Check sheet for the drawn part. Datum: minimum x, y, z corner. Units: mm. A direction names the side the tool comes from. Give positions to 0.01 mm unless a question says otherwise; leave off trailing zeros. Order: outer loops, then holes, each group sorted by start corner. A loop starts at its lowest first (then second) coordinate and runs counter-clockwise, first axis right, second up.
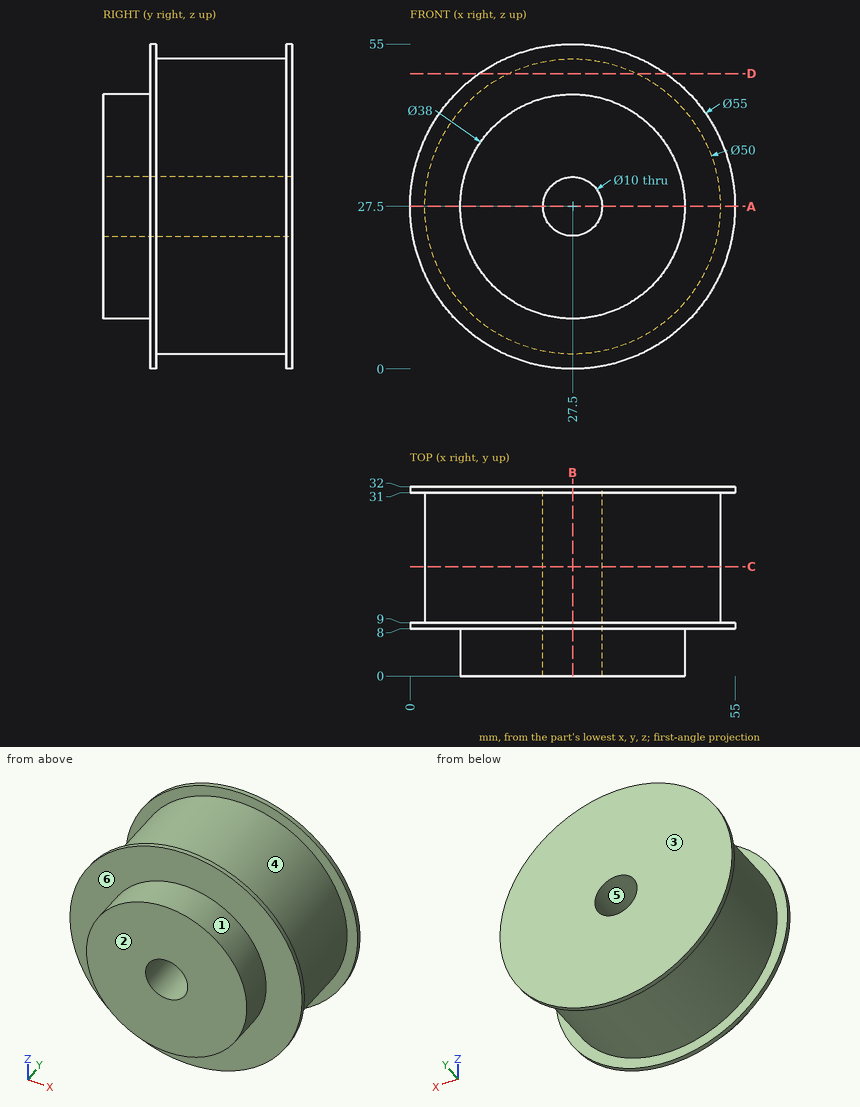
Item 1: Gauge pin test, flat ends, axial feed: pin 1 (8 mm diameter, centred on x = 44.5, z = 9, fed in from -Y); pin 2 (4 mm diameter, centred on x = 28, y = 5.5, fed in from +Z); pin 3 (1.5 mm diameter, centred on x = 44.5, y = 13.5, fed in from -Z); pin 4 (8 mm diameter, centred on x = 27.5, z = 27.5, fed in from +Y). Record the tip position at first contact, or that the pin passes through.
Reported:
pin 1: stops at y = 8
pin 2: stops at z = 46.5
pin 3: stops at z = 8.5
pin 4: passes through
Item 2: Set-up check for the marked faces 5 and 6: record each of +Z, -Z, +X, -X, +Y, -Y from which the full face is reachable in a straight line by a thin tool's end or side.
Reported:
face 5: +Y, -Y
face 6: -Y
Item 3: Sectioned sample at B-B (x = 27.5). Enter the section's corners in (y, z), and give its area (3 significant figures).
Reported:
outline: (0, 8.5) - (8, 8.5) - (8, 0) - (9, 0) - (9, 2.5) - (31, 2.5) - (31, 0) - (32, 0) - (32, 22.5) - (0, 22.5) - close; (0, 32.5) - (32, 32.5) - (32, 55) - (31, 55) - (31, 52.5) - (9, 52.5) - (9, 55) - (8, 55) - (8, 46.5) - (0, 46.5) - close
area: 1,190 mm2
Item 4: Scan lines: L1, parallel to Y at x = 51, z = 40.5; L2, parallel to X at y = 16, z = 27.5; L3, parallel to Y at x = 16, z = 5.5. Record each from-to range of solid material in increasing order.
Reported:
L1: y = 8 to 9, 31 to 32
L2: x = 2.5 to 22.5, 32.5 to 52.5
L3: y = 8 to 32
Item 5: Sectioned sample at A-A (z = 27.5). Enter the section's corners in (x, y), and give its area (3 significant figures).
Reported:
outline: (0, 8) - (8.5, 8) - (8.5, 0) - (22.5, 0) - (22.5, 32) - (0, 32) - (0, 31) - (2.5, 31) - (2.5, 9) - (0, 9) - close; (32.5, 0) - (46.5, 0) - (46.5, 8) - (55, 8) - (55, 9) - (52.5, 9) - (52.5, 31) - (55, 31) - (55, 32) - (32.5, 32) - close
area: 1,190 mm2
Item 6: Sectioned sample at D-D (z = 50). Enter the section's corners in (x, y).
Reported:
outline: (11.69, 8) - (43.31, 8) - (43.31, 9) - (38.4, 9) - (38.4, 31) - (43.31, 31) - (43.31, 32) - (11.69, 32) - (11.69, 31) - (16.6, 31) - (16.6, 9) - (11.69, 9) - close
Item 7: Sectioned sample at C-C (y = 18.5). Enter the section's corners in (x, z).
Reported:
outline: circle Ø50 at (27.5, 27.5); hole circle Ø10 at (27.5, 27.5)
Item 8: Draft check along Y on the marked faces 1, 2, 3 and 4. Enter one of: released by +Y, released by -Y, zero draft, split by the parting line, or undercut.
Reported:
face 1: zero draft
face 2: released by -Y
face 3: released by +Y
face 4: undercut
